from build123d import *

# Parameters (mm, degrees)
SKETCH146_R  = 1.9
PAD114_DEPTH = 3


with BuildPart() as innerbearingrace:
    # Sketch144 → Revolution005 (revolve)
    with BuildSketch(Plane(origin=(50, 160, -10), x_dir=(1, 0, 0), z_dir=(0, -1, 0))):
        Polygon((4.423355, 2), (3.02294, 0), (1.8, 0), (1.8, 2), align=None)
    revolve(axis=Axis((50, 160, -10), (0, 0, 1)))


with BuildPart() as steeringrod_long:
    # Sketch146 → Pad114 (new body)
    with BuildSketch(Plane(origin=(50, 160, -8), x_dir=(1, 0, 0), z_dir=(0, 0, 1))):
        with BuildLine():
            Line((9, 3.5), (2.828427, 3.5))
            ThreePointArc((2.828427, 3.5), (0, 4.5), (-2.828427, 3.5))
            Line((-2.828427, 3.5), (-8, 3.5))
            Line((-8, 3.5), (-8, -3.5))
            Line((-8, -3.5), (-2.828427, -3.5))
            ThreePointArc((-2.828427, -3.5), (0, -4.5), (2.828427, -3.5))
            Line((2.828427, -3.5), (9, -3.5))
            Line((9, -2.5), (9, -3.5))
            Line((12, -2.5), (9, -2.5))
            Line((12, 2.5), (12, -2.5))
            Line((9, 2.5), (12, 2.5))
            Line((9, 3.5), (9, 2.5))
        make_face()
        Circle(SKETCH146_R, mode=Mode.SUBTRACT)
    extrude(amount=PAD114_DEPTH)

    # Fusion004020022: union InnerBearingRace
    add(innerbearingrace.part)


solid = steeringrod_long.part
CAD build for the part. Positions are in the model's coordinates, mm. A direction names the side the tool comes from. Round coordinates to 2 decimals unless told otherwise and drop trailing zeros. Loops run counter-clockwise (first coordinate to the right, second up) from the corner with the lowest first, then second, coordinate; pieces in that order, holes last. Notation, with made-up numbers: M -3.5,79 L 29.5,79 A32 cw 29.5,112 Z; hole C 68.5,41.25 d9. An arc over 180 degrees is marked long. One line per question, with ' | ' between items. Start each with the question number.
Item 1: Pin check, flat tips, straight feed: pin 1 Ø1.5 at (x, z) = (60, -6) entering from +Y; pin 2 Ø0.5 at (y, z) = (163, -6.5) entering from +X; pin 3 Ø2.5 at (x, y) = (50, 160) entering from +Z; pin 4 Ø1.5 at (x, z) = (43.5, -6.5) entering from +Y. Stop position of each tip, or through.
Item 2: Cut at B-B, the plane x = 50. Write the cut outline in (y, z), plus the area to 3 significant figures.
Item 3: Which spindle directions (+Z, -Z, +X, -X, +Y, -Y) get a long thin tool onto all of the face, cutting with end or side? Do faces 1 (the flat face through (45, 163.5, -7)), 2 (the flat face through (61, 157.5, -7)), 3 (the flat face through (56, 163.5, -7)). Say none if no direction does.
Item 4: Cut at A-A, the plane y = 160. Write the cut outline in (x, z).
Item 5: Wall check: line 1 (Y direction, x = 50, z = -7.1); line 2 (X direction, y = 160, z = -6.5); line 3 (X direction, y = 159, z = -7.7). Give the ranges that are in metal, low to high.
Item 6: Cut at D-D, the plane x = 44. Write the cut outline in (y, z), plus the area to 3 significant figures.
Item 7: Cut at C-C, the plane z = -7.6. Write the cut outline in (x, y), plus the area to 3 significant figures.
Item 8: Two-plate mould, pull along X, no slides. Class faces 4 (the cylindrical face through (51.812, 160.571, -6.521)), 5 (the flat face through (52, 161, -5)), 6 (the cylindrical face through (49.61, 158.243, -8.986)), 7 (the cylindrical face through (50, 164.5, -6.5)): pulls with the +X half, pulls with the -X half, needs draft (parallel to the pull), parting line crosses it, or undercut.
Responses:
1) pin 1: stops at y = 162.5 | pin 2: stops at x = 59 | pin 3: passes through | pin 4: stops at y = 163.5
2) outline: M 155.5,-8 L 155.58,-8 L 156.98,-10 L 158.2,-10 L 158.2,-8 L 158.1,-8 L 158.1,-5 L 155.5,-5 Z; M 161.8,-10 L 163.02,-10 L 164.42,-8 L 164.5,-8 L 164.5,-5 L 161.9,-5 L 161.9,-8 L 161.8,-8 Z | area: 23.3 mm²
3) face 1: +Z, -Z, -X, +Y | face 2: +Z, -Z, +X, -Y | face 3: +Z, -Z, +X, +Y
4) outline: M 42,-8 L 45.58,-8 L 46.98,-10 L 48.2,-10 L 48.2,-8 L 48.1,-8 L 48.1,-5 L 42,-5 Z; M 51.8,-10 L 53.02,-10 L 54.42,-8 L 62,-8 L 62,-5 L 51.9,-5 L 51.9,-8 L 51.8,-8 Z
5) line 1: y = 155.5 to 158.1, 161.9 to 164.5 | line 2: x = 42 to 48.1, 51.9 to 62 | line 3: x = 42 to 48.38, 51.62 to 62
6) outline: M 156.5,-8 L 163.5,-8 L 163.5,-5 L 156.5,-5 Z | area: 21.0 mm²
7) outline: M 42,156.5 L 47.17,156.5 A4.5 ccw 52.83,156.5 L 59,156.5 L 59,157.5 L 62,157.5 L 62,162.5 L 59,162.5 L 59,163.5 L 52.83,163.5 A4.5 ccw 47.17,163.5 L 42,163.5 Z; hole C 50,160 d3.8 | area: 130 mm²
8) face 4: undercut | face 5: needs draft | face 6: undercut | face 7: parting line crosses it
